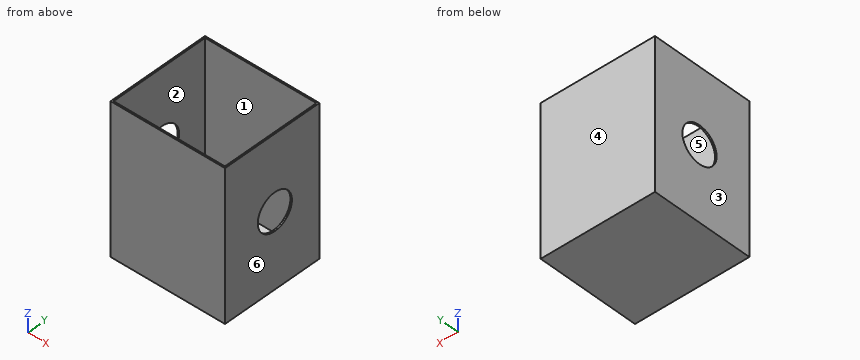
from build123d import *

# Parameters (mm, degrees)
F0_W     = 117.313064
F0_H     = 105.121065
F1_DEPTH = 152.4
F2_T     = -1.5875
F4_D     = 38.1


with BuildPart() as f1:
    # F0 (on Top) → F1 (new body)
    with BuildSketch(Plane.XY):
        with Locations((-9.687949, -2.982347)):
            Rectangle(F0_W, F0_H)
    extrude(amount=F1_DEPTH)

    # F2
    f2_openings = [f1.faces().sort_by_distance(p)[0] for p in [
        (-9.687949, -2.982346, 152.4),
    ]]
    offset(amount=F2_T, openings=f2_openings)

    # F4 (through all)
    with Locations(Plane.YZ.offset(48.968583)):
        with Locations((0, 76.2)):
            Hole(F4_D / 2)


solid = f1.part
Work out the finished part from the listing and answer in its coordinate system (mm). Face numbers are marked on the shaded views. A direction names the side the tool comes from. Give positions to 0.01 mm unless a question says otherwise; leave off trailing zeros. Order: outer loops, then holes, each group sorted by start corner. A loop starts at its lowest first (then second) coordinate and runs counter-clockwise, first axis right, second up. Notation, with made-up numbers: (31.25, 75.25) -> (76.25, 75.25) arc R20 ccw to (76.25, 96.25) -> close; hole circle Ø4 at (56.25, -13.75). An arc over 180 degrees is marked (long way). Answer as a JSON object with one key per item and string values. Group by question number.
1. Consider line 1 along X through (y, z) = (-46, 25.5); line 2 along Z through (x, y) = (-67.15, 0); line 3 along Y through (x, z) = (-67, 76). Determine where each line is inside the solid, lowest interval first. Write a range as [from, to].
2. Section C-C on z = 106 is taken. Determine the outline of the cut face in (x, y), plus the area to 3 significant figures.
3. Section B-B on z = 76.2 is taken. Determine the outline of the cut face in (x, y).
4. Section D-D on x = 6 is taken. Determine the outline of the cut face in (y, z).
5. The mould has two halves that part along Y. Classify the marked faces 1, 2, 3 and 4: released by +Y, released by -Y, zero draft, split by the parting line, or undercut.
6. Section A-A on y = 0 is taken. Determine the outline of the cut face in (x, z), plus the area to 3 significant figures.
7. Flat-ended cylindrical pins translate along their axes: pin 1 Ø1 at (x, y) = (29, 10) entering from -Z; pin 2 Ø2 at (x, y) = (23.5, -40) entering from +Z. Find the tip coordinate at first contact, or state that the pin passes through.
8. A tool of negligible diameter and unlimited length cuts with its end or side. For the marked faces 5 and 6, from which of +Z, -Z, +X, -X, +Y, -Y can it reach the whole face along a straight path? Write none if from no direction.
Result sheet:
{
 "1": {"line 1": "x = [-68.34, -66.76], [47.38, 48.97]", "line 2": "z = [0, 57.15], [95.25, 152.4]", "line 3": "y = [-55.54, -19.05], [19.05, 49.58]"},
 "2": {"outline": "(-68.34, -55.54) -> (48.97, -55.54) -> (48.97, 49.58) -> (-68.34, 49.58) -> close; hole (-66.76, -53.96) -> (47.38, -53.96) -> (47.38, 47.99) -> (-66.76, 47.99) -> close", "area": "696 mm^2"},
 "3": {"outline": "(-68.34, -55.54) -> (48.97, -55.54) -> (48.97, -19.05) -> (47.38, -19.05) -> (47.38, -53.96) -> (-66.76, -53.96) -> (-66.76, -19.05) -> (-68.34, -19.05) -> close; (-68.34, 19.05) -> (-66.76, 19.05) -> (-66.76, 47.99) -> (47.38, 47.99) -> (47.38, 19.05) -> (48.97, 19.05) -> (48.97, 49.58) -> (-68.34, 49.58) -> close"},
 "4": {"outline": "(-55.54, 0) -> (49.58, 0) -> (49.58, 152.4) -> (47.99, 152.4) -> (47.99, 1.59) -> (-53.96, 1.59) -> (-53.96, 152.4) -> (-55.54, 152.4) -> close"},
 "5": {"face 1": "undercut", "face 2": "undercut", "face 3": "zero draft", "face 4": "released by +Y"},
 "6": {"outline": "(-68.34, 0) -> (48.97, 0) -> (48.97, 57.15) -> (47.38, 57.15) -> (47.38, 1.59) -> (-66.76, 1.59) -> (-66.76, 57.15) -> (-68.34, 57.15) -> close; (-68.34, 95.25) -> (-66.76, 95.25) -> (-66.76, 152.4) -> (-68.34, 152.4) -> close; (47.38, 95.25) -> (48.97, 95.25) -> (48.97, 152.4) -> (47.38, 152.4) -> close", "area": "544 mm^2"},
 "7": {"pin 1": "stops at z = 0", "pin 2": "stops at z = 1.59"},
 "8": {"face 5": "+Z", "face 6": "+Z, -Z, +X, +Y, -Y"}
}
